The model under review builds one solid part; all positions refer to its coordinate system, in mm. Face numbers are marked on the shaded views. A direction names the side the tool comes from. Round coordinates to 2 decimals unless told otherwise and drop trailing zeros. Order: outer loops, then holes, each group sorted by start corner. A loop starts at its lowest first (then second) coordinate and runs counter-clockwise, first axis right, second up.
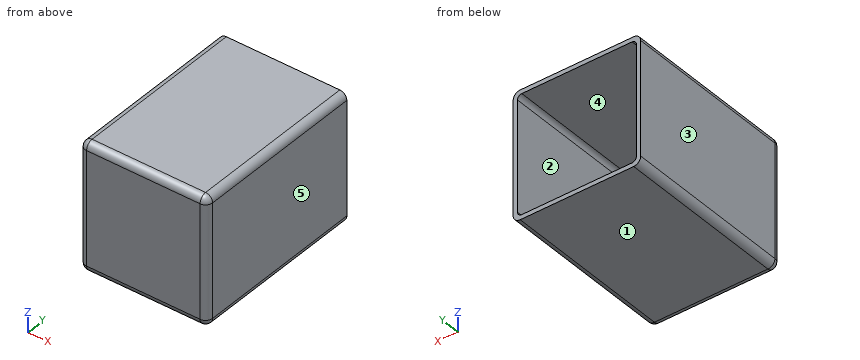
from build123d import *

# Parameters (mm, degrees)
SKETCH1_W           = 118
SKETCH1_H           = 118
BOSS_EXTRUDE1_DEPTH = 165
SHELL1_T            = -4
FILLET1_R           = 4
FILLET2_R           = 6.5


with BuildPart() as part:
    # Sketch1 → Boss-Extrude1 (new body)
    with BuildSketch(Plane(origin=(0, 0, 0), x_dir=(1, 0, 0), z_dir=(0, 1, 0))):
        Rectangle(SKETCH1_W, SKETCH1_H)
    extrude(amount=BOSS_EXTRUDE1_DEPTH)

    # Shell1
    shell1_openings = [part.faces().sort_by_distance(p)[0] for p in [
        (0, 165, 0),
    ]]
    offset(amount=SHELL1_T, openings=shell1_openings, kind=Kind.INTERSECTION)

    # Fillet1
    fillet1_edges = [part.edges().sort_by_distance(p)[0] for p in [
        (55, 4, 0),
        (55, 84.5, 55),
        (0, 4, -55),
        (55, 84.5, -55),
        (-55, 4, 0),
        (-55, 84.5, -55),
        (0, 4, 55),
        (-55, 84.5, 55),
    ]]
    fillet(fillet1_edges, radius=FILLET1_R)

    # Fillet2
    fillet2_edges = [part.edges().sort_by_distance(p)[0] for p in [
        (0, 0, 59),
        (-59, 0, 0),
        (0, 0, -59),
        (59, 0, 0),
        (59, 82.5, 59),
        (-59, 82.5, 59),
        (-59, 82.5, -59),
        (59, 82.5, -59),
    ]]
    fillet(fillet2_edges, radius=FILLET2_R)


solid = part.part
(1) We need section C-C (z = -36). Give the boundary of the cut face in (x, y), and give its area (3 significant figures).
(2) We need section B-B (y = 88.5). Give the boundary of the cut face in (x, z), and give its area (3 significant figures).
(3) Tool access review of the marked faces 4 and 5: name each direction out of +Z, -Z, +X, -X, +Y, -Y from which nothing blocks a thin tool from reaching the whole face with its end or side.
(4) We need section A-A (x = 7). Give the boundary of the cut face in (y, z).
(5) The part is to be moulded in two halves that separate along X. For the marked faces 1, 2 and 3, say which applies: pulls with the +X half, pulls with the -X half, needs draft (parallel to the pull), parting line crosses it, or undercut.
(6) Clearance check with a flat-ended pin moving along its axis: P1, Ø4, axis at x = -31, z = 7.5, coming from the +Y side. State where the tip first meets the part, or that it passes through.
(7) To check wall thickness, follow L1, parallel to Z at x = -40.5, y = 35.5; L2, parallel to Y at x = 33, z = -7.5. State the ranges of each line that lie inside material, in increasing order.
Verdict:
1. outline: (-59, 6.5) arc R6.5 ccw to (-52.5, 0) - (52.5, 0) arc R6.5 ccw to (59, 6.5) - (59, 165) - (55, 165) - (55, 8) arc R4 cw to (51, 4) - (-51, 4) arc R4 cw to (-55, 8) - (-55, 165) - (-59, 165) - close
1. area: 1,750 mm2
2. outline: (-59, -52.5) arc R6.5 ccw to (-52.5, -59) - (52.5, -59) arc R6.5 ccw to (59, -52.5) - (59, 52.5) arc R6.5 ccw to (52.5, 59) - (-52.5, 59) arc R6.5 ccw to (-59, 52.5) - close; hole (-55, -51) arc R4 ccw to (-51, -55) - (51, -55) arc R4 ccw to (55, -51) - (55, 51) arc R4 ccw to (51, 55) - (-51, 55) arc R4 ccw to (-55, 51) - close
2. area: 1,800 mm2
3. face 4: +Y
3. face 5: +Z, -Z, +X, +Y, -Y
4. outline: (0, -52.5) arc R6.5 ccw to (6.5, -59) - (165, -59) - (165, -55) - (8, -55) arc R4 cw to (4, -51) - (4, 51) arc R4 cw to (8, 55) - (165, 55) - (165, 59) - (6.5, 59) arc R6.5 ccw to (0, 52.5) - close
5. face 1: needs draft
5. face 2: undercut
5. face 3: pulls with the -X half
6. P1: stops at y = 4
7. L1: z = -59 to -55, 55 to 59
7. L2: y = 0 to 4
